For this review, take the finished solid that the model builds, in its own axes (mm). Give positions to 0.01 mm unless a question says otherwise; leave off trailing zeros. Write each loop counter-clockwise with the first axis right and the second up, starting at its lowest first coordinate (ties: lowest second). Pieces come first, ordered by that corner, then holes. Notation, with made-up numbers: M 12,13 L 67,13 A25 ccw 67,33 Z; hole C -7,38 d8. An arc over 180 degrees is marked long. Use one line per item in the form item = value. Start each with the question number.
Q1. For probe 1 along X at (y, z) = (0, -1); probe 2 along X at (y, z) = (-36, -20); probe 3 along Y at (x, z) = (376, -36), list the stretches that pass through material, from the lowest coordinate up. Write a range as [from, to].
Q2. Consider section A-A on x = -161. Write out the cut boundary in (y, z).
Q3. Clearance check with flat-ended pins moving along their axes: pin 1 Ø1 at (x, y) = (295.5, 9) entering from +Z; pin 2 Ø5 at (x, y) = (-425, -29.5) entering from -Z. State where each tip first meets the part, or that it passes through.
```python
from build123d import *

# Parameters (mm, degrees)
STRUCTURAL_MEMBER1_DEPTH = 900
SKETCH12_R               = 4.7625
CUT_EXTRUDE1_DEPTH       = 454.210052427
CUT_EXTRUDE2_DEPTH       = 40
SKETCH16_R               = 4.7625
CUT_EXTRUDE3_DEPTH       = 454.210052526
SKETCH17_R               = 4.7625
CUT_EXTRUDE4_DEPTH       = 454.210052526


with BuildPart() as part:
    # Sketch11 → Structural Member1 (new body)
    with BuildSketch(Plane(origin=(-450, 0, 0), x_dir=(0, 0, -1), z_dir=(1, 0, 0))):
        with BuildLine():
            Line((0, -38.1), (0, 38.1))
            Line((0, 38.1), (38.0492, 38.1))
            Line((38.0492, 38.1), (38.0492, 35.942335136))
            ThreePointArc((38.0492, 35.942335136), (37.447280466, 34.300554363), (35.926803066, 33.436899509))
            Line((35.926803066, 33.436899509), (12.283671721, 29.496090157))
            ThreePointArc((12.283671721, 29.496090157), (8.178382741, 27.164222052), (6.5532, 22.731413966))
            Line((6.5532, 22.731413966), (6.5532, -22.731413966))
            ThreePointArc((6.5532, -22.731413966), (8.178382741, -27.164222052), (12.283671721, -29.496090157))
            Line((12.283671721, -29.496090157), (35.926803066, -33.436899509))
            ThreePointArc((35.926803066, -33.436899509), (37.447280466, -34.300554363), (38.0492, -35.942335136))
            Line((38.0492, -35.942335136), (38.0492, -38.1))
            Line((38.0492, -38.1), (0, -38.1))
        make_face()
    extrude(amount=STRUCTURAL_MEMBER1_DEPTH)

    # Sketch12 → Cut-Extrude1 (cut, through all)
    with BuildSketch(Plane(origin=(0, 0, 0), x_dir=(1, 0, 0), z_dir=(0, 1, 0))):
        with Locations(Location((-425, 20, 0), (0, 0, 270))):
            Circle(SKETCH12_R)
        with Locations(Location((425, 20, 0), (0, 0, 270))):
            Circle(SKETCH12_R)
    extrude(amount=-CUT_EXTRUDE1_DEPTH, mode=Mode.SUBTRACT)

    # Sketch15 → Cut-Extrude2 (cut)
    with BuildSketch(Plane(origin=(0, 0, -6.5532), x_dir=(-1, 0, 0), z_dir=(0, 0, -1))):
        with BuildLine():
            Line((-412.5, -33.1), (-437.5, -33.1))
            ThreePointArc((-437.5, -33.1), (-442.5, -28.1), (-437.5, -23.1))
            Line((-437.5, -23.1), (-412.5, -23.1))
            ThreePointArc((-412.5, -23.1), (-407.5, -28.1), (-412.5, -33.1))
        make_face()
        with BuildLine():
            Line((412.5, -33.1), (437.5, -33.1))
            ThreePointArc((437.5, -33.1), (442.5, -28.1), (437.5, -23.1))
            Line((437.5, -23.1), (412.5, -23.1))
            ThreePointArc((412.5, -23.1), (407.5, -28.1), (412.5, -33.1))
        make_face()
    extrude(amount=CUT_EXTRUDE2_DEPTH, mode=Mode.SUBTRACT)

    # Sketch16 → Cut-Extrude3 (cut, through all)
    with BuildSketch(Plane(origin=(0, 0, 0), x_dir=(1, 0, 0), z_dir=(0, 1, 0))):
        with Locations(Location((-215.6, 20, 0), (0, 0, 270))):
            Circle(SKETCH16_R)
        with Locations(Location((-179.8, 20, 0), (0, 0, 270))):
            Circle(SKETCH16_R)
        with Locations(Location((179.8, 20, 0), (0, 0, 90))):
            Circle(SKETCH16_R)
        with Locations(Location((215.6, 20, 0), (0, 0, 90))):
            Circle(SKETCH16_R)
        with Locations(Location((-245, 20, 0), (0, 0, 270))):
            Circle(SKETCH16_R)
        with Locations(Location((-280, 20, 0), (0, 0, 270))):
            Circle(SKETCH16_R)
        with Locations(Location((245, 20, 0), (0, 0, 90))):
            Circle(SKETCH16_R)
        with Locations(Location((280, 20, 0), (0, 0, 90))):
            Circle(SKETCH16_R)
    extrude(amount=CUT_EXTRUDE3_DEPTH, mode=Mode.SUBTRACT)

    # Sketch17 → Cut-Extrude4 (cut, through all)
    with BuildSketch(Plane.XY):
        with Locations((228.7, 0.6)):
            Circle(SKETCH17_R)
        with Locations((-228.7, 0.6)):
            Circle(SKETCH17_R)
    extrude(amount=-CUT_EXTRUDE4_DEPTH, mode=Mode.SUBTRACT)


solid = part.part
```
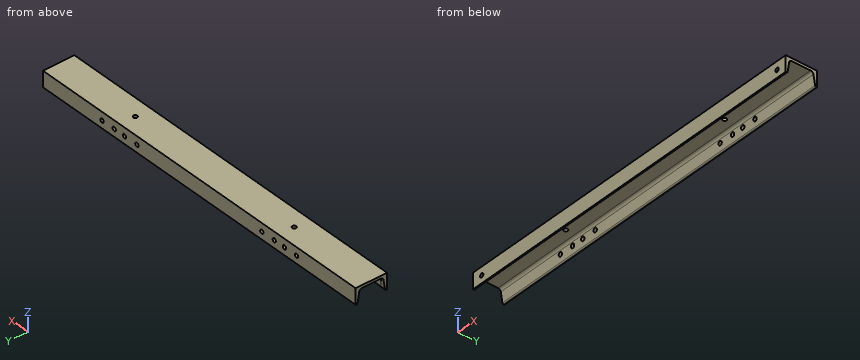
Working result:
q1.probe_1 = [-450, -233.42], [-223.98, 223.98], [233.42, 450]
q1.probe_2 = [-450, -429.76], [-420.24, 420.24], [429.76, 450]
q1.probe_3 = [-38.1, -33.45], [33.45, 38.1]
q2.outline = M -38.1,-38.05 L -35.94,-38.05 A2.54 ccw -33.44,-35.93 L -29.5,-12.28 A6.86 cw -22.73,-6.55 L 22.73,-6.55 A6.86 cw 29.5,-12.28 L 33.44,-35.93 A2.54 ccw 35.94,-38.05 L 38.1,-38.05 L 38.1,0 L -38.1,0 Z
q3.pin_1 = 0
q3.pin_2 = -6.55
